```python
from build123d import *

# Parameters (mm, degrees)
ESQUISSE2_R             = 10
BOSS_EXTRU_1_DEPTH      = 20
ENL_V_START             = -10
ESQUISSE3_R             = 11
ESQUISSE3_R_2           = 10
ENL_V_MAT_EXTRU_1_DEPTH = 10
ESQUISSE4_W             = 3
ESQUISSE4_H             = 10
BOSS_EXTRU_2_DEPTH      = 4
ESQUISSE5_R             = 1.1
BOSS_EXTRU_3_DEPTH      = 1
ESQUISSE9_R             = 1.1
BOSS_EXTRU_5_DEPTH      = 2
BOSS_EXTRU_6_START      = -6
BOSS_EXTRU_6_DEPTH      = 8
CONG_1_R                = 1
CONG_2_R                = 1


with BuildPart() as part:
    # Esquisse2 → Boss.-Extru.1 (new body)
    with BuildSketch(Plane.XY):
        with BuildLine():
            Line((5.727272727, 12.774910845), (24.045454545, 4.562468159))
            ThreePointArc((24.045454545, 4.562468159), (27, 0), (24.045454545, -4.562468159))
            Line((24.045454545, -4.562468159), (5.727272727, -12.774910845))
            ThreePointArc((5.727272727, -12.774910845), (-14, 0), (5.727272727, 12.774910845))
        make_face()
        Circle(ESQUISSE2_R, mode=Mode.SUBTRACT)
    extrude(amount=BOSS_EXTRU_1_DEPTH)

    # Esquisse3 → Enlèv. mat.-Extru.1 (cut)
    with BuildSketch(Plane.XY.offset(20).offset(ENL_V_START)):
        Circle(ESQUISSE3_R)
        Circle(ESQUISSE3_R_2, mode=Mode.SUBTRACT)
    extrude(amount=ENL_V_MAT_EXTRU_1_DEPTH, mode=Mode.SUBTRACT)

    # Esquisse4 → Boss.-Extru.2 (add)
    with BuildSketch(Plane(origin=(5.727272727, -12.774910845, 0), x_dir=(0.9124936318129423, 0.4090909090909094, 0), z_dir=(0.40909090909090934, -0.9124936318129422, 0))):
        with Locations((17.5748599, 10)):
            Rectangle(ESQUISSE4_W, ESQUISSE4_H)
    extrude(amount=BOSS_EXTRU_2_DEPTH)

    # Esquisse5 → Boss.-Extru.3 (add)
    with BuildSketch(Plane.XY.offset(15)):
        with Locations(Location((22.582402284, -7.410182695, 0), (0, 0, 180))):
            Circle(ESQUISSE5_R)
    boss_extru_3 = extrude(amount=BOSS_EXTRU_3_DEPTH)

    # Symétrie1: Boss.-Extru.3 across plane
    add(boss_extru_3.mirror(Plane.XY.offset(10)))

    # Esquisse9 → Boss.-Extru.5 (add)
    # profile 1 of 2: a face of its own
    with BuildSketch(Plane.XY.offset(16)):
        with BuildLine():
            Line((21.323895477, -10.714144048), (23.605129557, -9.691416775))
            ThreePointArc((23.605129557, -9.691416775), (24.737785683, -6.717851558), (21.764220466, -5.585195432))
            Line((21.764220466, -5.585195432), (19.482986386, -6.607922705))
            Line((19.482986386, -6.607922705), (21.323895477, -10.714144048))
        make_face()
        with Locations(Location((22.582402284, -7.410182695, 0), (0, 0, 180))):
            Circle(ESQUISSE9_R, mode=Mode.SUBTRACT)
    # profile 2 of 2: a face of its own
    with BuildSketch(Plane.XY.offset(16)):
        with Locations(Location((22.582402284, -7.410182695, 0), (0, 0, 180))):
            Circle(ESQUISSE9_R)
    boss_extru_5 = extrude(amount=BOSS_EXTRU_5_DEPTH)

    # Esquisse9<4> → Boss.-Extru.6 (add)
    with BuildSketch(Plane.XY.offset(16).offset(BOSS_EXTRU_6_START)):
        with BuildLine():
            Line((-2.260153649, -21.287390546), (21.323895477, -10.714144048))
            Line((21.323895477, -10.714144048), (19.482986386, -6.607922705))
            Line((19.482986386, -6.607922705), (1.283727254, -14.767049742))
            ThreePointArc((1.283727254, -14.767049742), (0.201847525, -15.178661138), (-0.920349818, -15.462493505))
            Line((-0.920349818, -15.462493505), (-5.484659611, -16.339454049))
            ThreePointArc((-5.484659611, -16.339454049), (-7.55515779, -21.213423405), (-2.260153649, -21.287390546))
        make_face()
    boss_extru_6 = extrude(amount=BOSS_EXTRU_6_DEPTH)

    # Symétrie2: Boss.-Extru.5, Boss.-Extru.6 across plane
    add(boss_extru_5.mirror(Plane.XY.offset(10)))
    add(boss_extru_6.mirror(Plane.XY.offset(10)))

    # Congé1
    cong_1_edges = [part.edges().sort_by_distance(p)[0] for p in [
        (24.76932455, -8.621533595, 10),
    ]]
    fillet(cong_1_edges, radius=CONG_1_R)

    # Congé2
    cong_2_edges = [part.edges().sort_by_distance(p)[0] for p in [
        (22.031843655, -9.848806323, 10),
    ]]
    fillet(cong_2_edges, radius=CONG_2_R)


solid = part.part
```
Here's how the part is built. I have some questions about the finished solid (model axes, mm). A direction names the side the tool comes from. Coordinates: 2 decimals unless noted, no trailing zeros. Order: outer loops, then holes, each group sorted by start corner. A loop starts at its lowest first (then second) coordinate and runs counter-clockwise, first axis right, second up. Notation, with made-up numbers: M 34,-23 L 75,-23 A17 ccw 75,-13 Z; hole C 15.5,-6 d7. An arc over 180 degrees is marked long. Answer as a JSON object with one key per item and string values. Group by question number.
(1) Which directions (+Z, -Z, +X, -X, +Y, -Y) give clear straight access to the entire face, cutting with the end or side of a thin tool? Please do faces 1 (the face through (21, -7, 15)), 2 (the face through (7, -14, 2)), 3 (the face through (23.39, -9.24, 10.07)), 4 (the face through (-2.38, -10.74, 14.93)).
(2) For pin 1 (2.5 mm diameter, centred on x = 21.5, y = -8.5, fed in from -Z); pin 2 (1 mm diameter, centred on y = -9, z = 8.5, fed in from +X); pin 3 (5 mm diameter, centred on x = 12.5, y = -14, fed in from +Z), each with a flat end and sliding along its axis, tell me the tip position at first contact or that it passes through.
(3) Suppose I cut it at B-B, the plane z = 13. Please give me the cut outline in (x, y), then the cut area to 3 significant figures.
(4) If we mould it in two halves opening along X, with no side actions, what happens to faces 5 (the face through (11, 0, 0)), 6 (the face through (-7.6, -21.14, 10.11)), 7 (the face through (22, -9, 4)), 8 (the face through (23.738, -6.321, 9.93))? For each: released by +X, released by -X, zero draft, split by the parting line, or undercut.
(5) Suppose I cut it at C-C, the plane x = 0. Please give me the cut outline in (y, z), then the cut area to 3 significant figures.
(6) I need wall thicknesses on probe 1 along Y at (x, z) = (0, 15.25); probe 2 along Y at (x, z) = (3.5, 7); probe 3 along X at (y, z) = (4.5, 16). Which ranges of each line are inside material? Lowest first, please.
(7) Suppose I cut it at A-A, the plane y = 0. Please give me the cut outline in (x, z), then the cut area to 3 significant figures.
(8) Suppose I cut it at D-D, the plane x = 9. Please give me the cut outline in (y, z).
Values found:
{
 "1": {"face 1": "none", "face 2": "-Z, +X, -Y", "face 3": "+X, -Y", "face 4": "+Z"},
 "2": {"pin 1": "stops at z = 2", "pin 2": "stops at x = 24.37", "pin 3": "stops at z = 18"},
 "3": {"outline": "M -5.48,-16.34 A3.19 ccw long -2.26,-21.29 L 21.32,-10.71 L 19.48,-6.61 L 20.4,-6.2 L 21.62,-8.94 A1 ccw 22.94,-9.44 L 23.86,-9.03 A1 ccw 24.36,-7.71 L 23.13,-4.97 L 24.05,-4.56 A5 ccw 24.05,4.56 L 5.73,12.77 A14 ccw long 5.73,-12.77 L 1.28,-14.77 A10 cw -0.92,-15.46 Z; hole C 0,0 d22", "area": "577 mm^2"},
 "4": {"face 5": "zero draft", "face 6": "split by the parting line", "face 7": "undercut", "face 8": "released by +X"},
 "5": {"outline": "M -20.27,2 L -15.24,2 L -15.24,18 L -20.27,18 Z; M -14,0 L -10,0 L -10,10 L -11,10 L -11,20 L -14,20 Z; M 10,0 L 14,0 L 14,20 L 11,20 L 11,10 L 10,10 Z", "area": "221 mm^2"},
 "6": {"probe 1": "y = -20.27 to -15.24, -14 to -11, 11 to 14", "probe 2": "y = -18.7 to -13.77, -13.56 to -9.37, 9.37 to 13.56", "probe 3": "x = -13.26 to -10.04, 10.04 to 24.18"},
 "7": {"outline": "M -14,0 L -10,0 L -10,10 L -11,10 L -11,20 L -14,20 Z; M 10,0 L 27,0 L 27,20 L 11,20 L 11,10 L 10,10 Z", "area": "400 mm^2"},
 "8": {"outline": "M -16.24,2 L -11.31,2 L -11.31,0 L -4.36,0 L -4.36,10 L -6.32,10 L -6.32,20 L -11.31,20 L -11.31,18 L -16.24,18 Z; M 4.36,0 L 11.31,0 L 11.31,20 L 6.32,20 L 6.32,10 L 4.36,10 Z"}
}
